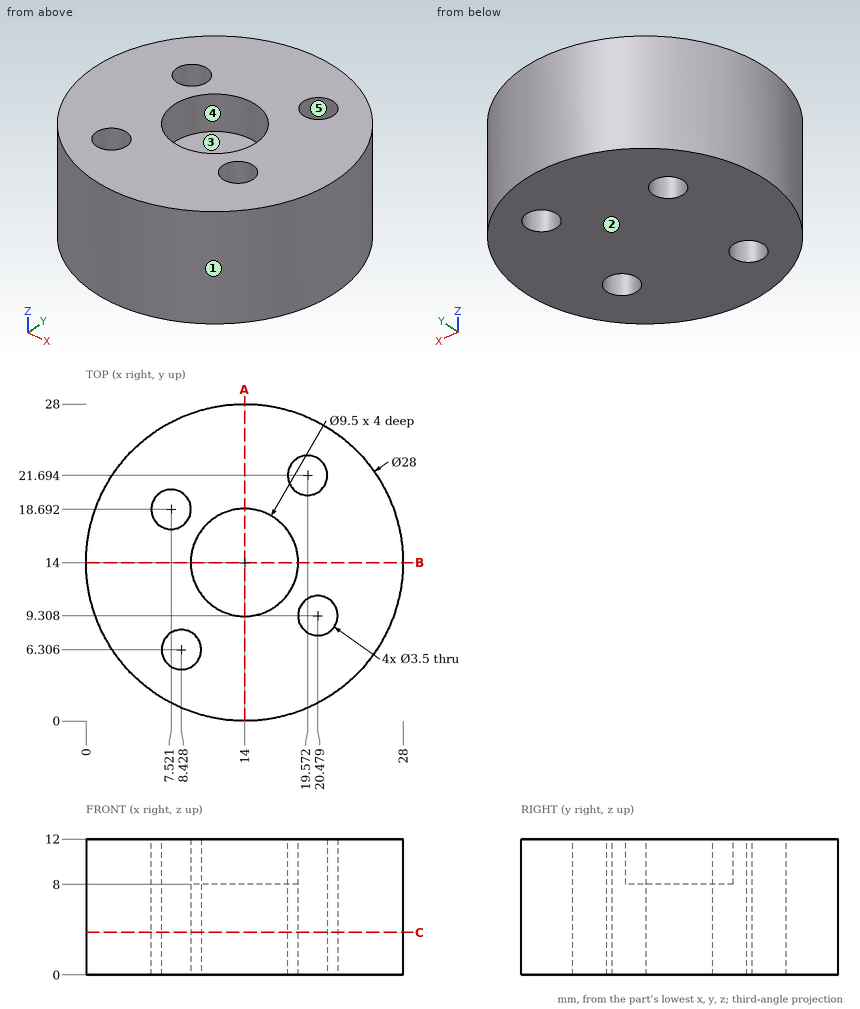
Source: three-view drawing plus pictorial views. Frame: mm from the lowest corner of the part. A direction names the side the tool comes from. Coordinates: 2 decimals unless noted, no trailing zeros. Loops run counter-clockwise (first coordinate to the right, second up) from the corner with the lowest first, then second, coordinate; pieces in that order, holes last. Notation, with made-up numbers: (8.25, 70) -> (21.25, 70) arc R18 cw to (21.25, 91) -> close; hole circle Ø1 at (-4.5, 31.25). An arc over 180 degrees is marked (long way). Answer in a Markdown table with one row per item. Add a question column.
Q1. Contact query for flat-ended pins moving along their axis: pin 1 Ø1 at (x, y) = (9, 7) entering from -Z; pin 2 Ø5 at (y, z) = (7.5, 4.5) entering from +X; pin 3 Ø5 at (y, z) = (18.5, 7.5) entering from +X; pin 4 Ø1.5 at (y, z) = (6, 4) entering from +X. Output: stop coordinate, or through.
Q2. Pull-direction query (X, two-part tool) for the marked faces 1, 2 and 3; classes: pulls with the +X half, pulls with the -X half, needs draft (parallel to the pull), parting line crosses it, or undercut.
Q3. Ray query, line 1 along X through (y, z) = (7.75, 3) (1 decimal); line 2 along Y through (x, z) = (13.75, 8.25); line 3 along Y through (x, z) = (7.75, 7.5). Return the intervals inside material, ascending.
Q4. Reachability of the marked faces 4 and 5 from +Z, -Z, +X, -X, +Y, -Y: full face, straight path, thin tool, end or side. Return the list, or none.
Q5. Section A-A on x = 14. Return the cut outline in (y, z), and give its area (3 significant figures).
Q6. Section C-C on z = 3.75. Give the number of separate pieces and of enclosed holes in the cut face, and give its area (3 significant figures).
Computed values:
| question | item | result |
|---|---|---|
| 1 | pin 1 | passes through |
| 1 | pin 2 | stops at x = 27.42 |
| 1 | pin 3 | stops at x = 27.86 |
| 1 | pin 4 | stops at x = 25.98 |
| 2 | face 1 | parting line crosses it |
| 2 | face 2 | needs draft |
| 2 | face 3 | undercut |
| 3 | line 1 | x = 1.5 to 7.4, 9.4 to 19.7, 21.3 to 26.5 |
| 3 | line 2 | y = 0 to 9.26, 18.74 to 28 |
| 3 | line 3 | y = 1.47 to 4.69, 7.92 to 16.96, 20.43 to 26.53 |
| 4 | face 4 | +Z |
| 4 | face 5 | +Z, -Z |
| 5 | outline | (0, 0) -> (28, 0) -> (28, 12) -> (18.75, 12) -> (18.75, 8) -> (9.25, 8) -> (9.25, 12) -> (0, 12) -> close |
| 5 | area | 298 mm^2 |
| 6 | separate pieces | 1 |
| 6 | enclosed holes | 4 |
| 6 | area | 577 mm^2 |
